For this review, take the finished solid that the model builds, in its own axes (mm). Face numbers are marked on the shaded views. A direction names the side the tool comes from. Coordinates: 2 decimals unless noted, no trailing zeros. Write each loop counter-clockwise with the first axis right and the second up, starting at its lowest first coordinate (ties: lowest second). Pieces come first, ordered by that corner, then holes.
1) To check wall thickness, follow line 1 along X through (y, z) = (2.25, 25); line 2 along Z through (x, y) = (32.5, 3.5); line 3 along X through (y, z) = (4.5, -10). State the ranges of each line that lie inside material, in increasing order.
2) We need section A-A on x = -10.5. Write out the cut boundary in (y, z), then the cut area to 4 significant figures.
3) Insertion check: P1, Ø3, axis at x = 32.5, z = 25, coming from the +Y side. The pin has a flat end and moves straight along its axis. Give the tip position at first contact, or say it passes through.
4) We need section C-C on z = 12. Write out the cut boundary in (x, y), then the cut area to 3 significant figures.
5) We need section D-D on z = 25. Write out the cut boundary in (x, y).
6) Mouldability with a two-part tool opening along X and no side actions: class the marked faces 3, 4 and 5 as pulls with the +X half, pulls with the -X half, needs draft (parallel to the pull), parting line crosses it, or undercut.
7) We need section B-B on x = 32.5. Write out the cut boundary in (y, z).
8) For the marked faces 1 and 2, list the 3-axis set-ups (+Z, -Z, +X, -X, +Y, -Y) from which the entire face can be reached by the end or side of a thin tool; tool diameter is ignored.
from build123d import *

# Parameters (mm, degrees)
BOSS_EXTRUDE1_DEPTH         = 6.35
TAP_DRILL_FOR_M5X0_8_TAP1_D = 3.5
SKETCH4_R                   = 10
CUT_EXTRUDE1_DEPTH          = 52.054603123


with BuildPart() as part:
    # Sketch1 → Boss-Extrude1 (new body)
    with BuildSketch(Plane(origin=(0, 0, 0), x_dir=(1, 0, 0), z_dir=(0, 1, 0))):
        with BuildLine():
            Line((34.5, -33.5), (-34.5, -33.5))
            ThreePointArc((-34.5, -33.5), (-36.974873734, -32.474873734), (-38, -30))
            Line((-38, -30), (-38, 30))
            ThreePointArc((-38, 30), (-36.974873734, 32.474873734), (-34.5, 33.5))
            Line((-34.5, 33.5), (34.5, 33.5))
            ThreePointArc((34.5, 33.5), (36.974873734, 32.474873734), (38, 30))
            Line((38, 30), (38, -30))
            ThreePointArc((38, -30), (36.974873734, -32.474873734), (34.5, -33.5))
        make_face()
        with BuildLine():
            Line((24.5, -29), (-24.5, -29))
            ThreePointArc((-24.5, -29), (-25.560660172, -28.560660172), (-26, -27.5))
            Line((-26, -27.5), (-26, 27.5))
            ThreePointArc((-26, 27.5), (-25.560660172, 28.560660172), (-24.5, 29))
            Line((-24.5, 29), (24.5, 29))
            ThreePointArc((24.5, 29), (25.560660172, 28.560660172), (26, 27.5))
            Line((26, 27.5), (26, -27.5))
            ThreePointArc((26, -27.5), (25.560660172, -28.560660172), (24.5, -29))
        make_face(mode=Mode.SUBTRACT)
    extrude(amount=BOSS_EXTRUDE1_DEPTH)

    # Tap Drill for M5x0.8 Tap1 (through all)
    with Locations(Plane(origin=(0, 6.35, 0), x_dir=(1, 0, 0), z_dir=(0, 1, 0))):
        with Locations((-32.5, -25), (-32.5, 25), (32.5, -25), (32.5, 25)):
            Hole(TAP_DRILL_FOR_M5X0_8_TAP1_D / 2)

    # Sketch4 → Cut-Extrude1 (cut, through all)
    with BuildSketch(Plane(origin=(0, 6.35, 0), x_dir=(1, 0, 0), z_dir=(0, 1, 0))):
        with Locations((0, -20)):
            Circle(SKETCH4_R)
    extrude(amount=-CUT_EXTRUDE1_DEPTH, mode=Mode.SUBTRACT)


solid = part.part
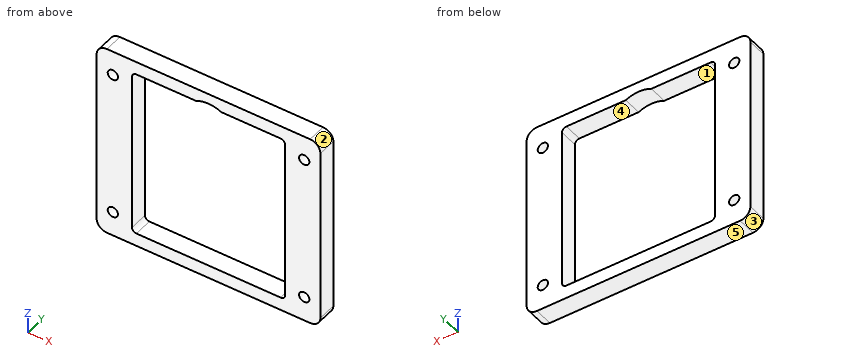
Result:
1. line 1: x = -38 to -34.25, -30.75 to -26, 26 to 30.75, 34.25 to 38
1. line 2: z = -33.5 to -26.75, -23.25 to 23.25, 26.75 to 33.5
1. line 3: x = -38 to -26, 26 to 38
2. outline: (0, -33.5) - (6.35, -33.5) - (6.35, -29) - (0, -29) - close; (0, 29) - (6.35, 29) - (6.35, 33.5) - (0, 33.5) - close
2. area: 57.15 mm2
3. P1: passes through
4. outline: (-38, 0) - (-26, 0) - (-26, 6.35) - (-38, 6.35) - close; (26, 0) - (38, 0) - (38, 6.35) - (26, 6.35) - close
4. area: 152 mm2
5. outline: (-38, 0) - (-34.25, 0) - (-34.25, 6.35) - (-38, 6.35) - close; (-30.75, 0) - (-26, 0) - (-26, 6.35) - (-30.75, 6.35) - close; (26, 0) - (30.75, 0) - (30.75, 6.35) - (26, 6.35) - close; (34.25, 0) - (38, 0) - (38, 6.35) - (34.25, 6.35) - close
6. face 3: pulls with the -X half
6. face 4: undercut
6. face 5: needs draft
7. outline: (0, -33.5) - (6.35, -33.5) - (6.35, -26.75) - (0, -26.75) - close; (0, -23.25) - (6.35, -23.25) - (6.35, 23.25) - (0, 23.25) - close; (0, 26.75) - (6.35, 26.75) - (6.35, 33.5) - (0, 33.5) - close
8. face 1: +Y, -Y
8. face 2: +Z, +X, +Y, -Y
